Autodesk Inventor part; units mm, degrees
ref_plane "YZ Plane" through (0, 0, 0) normal (1, 0, 0) x (0, 1, 0)
ref_plane "XZ Plane" through (0, 0, 0) normal (0, 1, 0) x (-1, 0, 0)
ref_plane "XY Plane" through (0, 0, 0) normal (0, 0, 1) x (1, 0, 0)
sketch "Sketch1" plane through (0, 0, 0) normal (1, 0, 0) x (0, 1, 0)
  line L0 (0, 0) -> (25.4, 0)
  line L1 (25.4, 0) -> (25.4, 38.1)
  line L2 (25.4, 38.1) -> (0, 38.1)
  line L3 (0, 38.1) -> (0, 0)
  dimension "d0" = 25.4
  dimension "d1" = 38.1
extrude "Extrusion1" add sketch "Sketch1" along normal blind 1.5875
sketch "Sketch2" plane through (1.5875, 0, 0) normal (1, 0, 0) x (0, 0, -1)
  line L0 (-38.1, 0) -> (0, 0)
  line L1 (0, 25.4) -> (-1.5875, 25.4)
  line L2 (-1.5875, 25.4) -> (-1.5875, 0)
  line L3 (-1.5875, 0) -> (0, 0)
  line L4 (0, 0) -> (0, 25.4)
  dimension "d4" = 1.5875
extrude "Extrusion2" add sketch "Sketch2" along normal blind 23.8125
sketch "Sketch3" plane through (1.5875, 0, 0) normal (1, 0, 0) x (0, 0, -1)
  line L0 (-1.5875, 25.4) -> (-38.1, 25.4)
  line L1 (-38.1, 25.4) -> (-38.1, 0)
  point P0 (0, 0)
  point P1 (-25.3973, 12.7)
  dimension "d8" = 12.7027
  dimension "d9" = 12.7
hole "Hole1" at (1.5875, 12.7, 25.3973) direction (-1, 0, 0) diameter 6.35 end through all
sketch "Sketch4" plane through (1.5875, 0, 1.5875) normal (0, 0, 1) x (1, 0, 0)
  line L0 (23.8125, 25.4) -> (23.8125, 0)
  line L1 (0, 25.4) -> (23.8125, 25.4)
  point P0 (-1.5875, 0)
  point P1 (11.1125, 12.7)
  dimension "d17" = 12.7
  dimension "d18" = 12.7
hole "Hole2" at (12.7, 12.7, 1.5875) direction (0, 0, -1) diameter 6.35 end through all
properties part number "LBrace" material "Aluminum 6061"
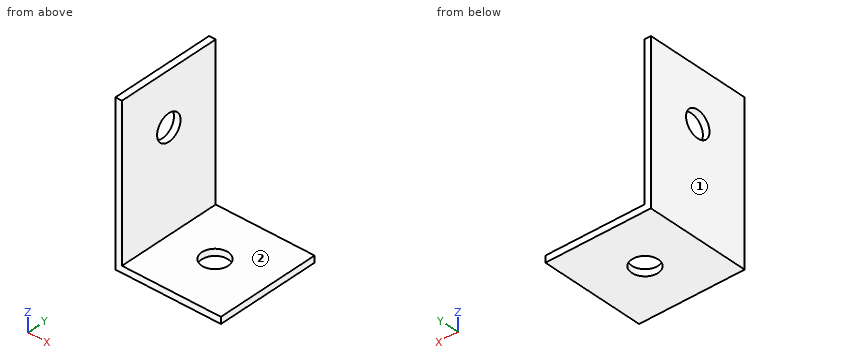
The model under review builds one solid part; all positions refer to its coordinate system, in mm. Face numbers are marked on the shaded views. A direction names the side the tool comes from. Round coordinates to 2 decimals unless told otherwise and drop trailing zeros. Loops run counter-clockwise (first coordinate to the right, second up) from the corner with the lowest first, then second, coordinate; pieces in that order, holes last. Notation, with made-up numbers: (36, -13.75) - (49, -13.75) arc R16 cw to (49, -0.75) - close; hole circle Ø7 at (-18.75, 33.5). An arc over 180 degrees is marked (long way). Use a Markdown table: item, result. Add a question column.
Q1. Add section B-B (x = 12.7). State the section outline as (y, z) points (1 decimal).
Q2. Add section D-D (y = 6). State the section outline as (x, z) points, plus the area to 3 significant figures.
Q3. For probe 1 along Z at (x, y) = (6, 7.5); probe 2 along X at (y, z) = (12.7, 0.7) (3 decimals), list the stretches that pass through material, from the lowest coordinate up.
Q4. Add section A-A (y = 12.7). State the section outline as (x, z) points (1 decimal), plus the area to 3 significant figures.
Q5. Insertion check: pin 1 Ø4 at (x, z) = (20.5, 4) entering from -Y (1 decimal); pin 2 Ø4 at (x, y) = (14.5, 13) entering from -Z; pin 3 Ø5 at (x, y) = (15.5, 6) entering from +Z; pin 4 Ø12 at (y, z) = (5, 33.5) entering from +X. Each pin has a flat end and moves straight along its axis. Give the tip position at first contact, or say it passes through.
Q6. Add section C-C (z = 17.5). State the section outline as (x, y) points.
Q7. Machinability: for the marked faces 1 and 2, which of the approach directions +Z, -Z, +X, -X, +Y, -Y give a long, thin tool a straight path to every point of the face, cutting with its end or side? Answer none if there is none.
Worked answers:
| question | item | result |
|---|---|---|
| 1 | outline | (0, 0) - (9.5, 0) - (9.5, 1.6) - (0, 1.6) - close; (15.9, 0) - (25.4, 0) - (25.4, 1.6) - (15.9, 1.6) - close |
| 2 | outline | (0, 0) - (25.4, 0) - (25.4, 1.59) - (1.59, 1.59) - (1.59, 38.1) - (0, 38.1) - close |
| 2 | area | 98.3 mm² |
| 3 | probe 1 | 0 to 1.59 |
| 3 | probe 2 | 0 to 9.525, 15.875 to 25.4 |
| 4 | outline | (0, 0) - (9.5, 0) - (9.5, 1.6) - (1.6, 1.6) - (1.6, 22.2) - (0, 22.2) - close; (0, 28.6) - (1.6, 28.6) - (1.6, 38.1) - (0, 38.1) - close; (15.9, 0) - (25.4, 0) - (25.4, 1.6) - (15.9, 1.6) - close |
| 4 | area | 78.1 mm² |
| 5 | pin 1 | through |
| 5 | pin 2 | z = 0 |
| 5 | pin 3 | z = 1.59 |
| 5 | pin 4 | x = 1.59 |
| 6 | outline | (0, 0) - (1.59, 0) - (1.59, 25.4) - (0, 25.4) - close |
| 7 | face 1 | +Z, -Z, -X, +Y, -Y |
| 7 | face 2 | +Z, +X, +Y, -Y |
